from build123d import *

# Parameters (mm, degrees)
SKETCH1_R              = 2.925
SKETCH1_R_2            = 1.75
MIDDLE_RING_DEPTH      = 0.8
SKETCH2_R              = 2.35
SKETCH2_R_2            = 1.75
OUTER_BODY_DEPTH       = 7.35
SKETCH3_R              = 2.625
SKETCH3_R_2            = 1.75
OUTER_RIM_DEPTH        = 0.5
MIDDLE_SLOT_DEPTH      = 9.873204044
MIDDLE_SLOT_DEPTH_BACK = 9.873204044
SIDE_SLOTS_DEPTH       = 9.859105574
SIDE_SLOTS_DEPTH_BACK  = 9.859105574


with BuildPart() as part:
    # Sketch1 → Middle Ring (new, symmetric)
    with BuildSketch(Plane(origin=(0, 0, 0), x_dir=(0, 0, -1), z_dir=(1, 0, 0))):
        Circle(SKETCH1_R)
        Circle(SKETCH1_R_2, mode=Mode.SUBTRACT)
    extrude(amount=MIDDLE_RING_DEPTH, both=True)

    # Sketch2 → Outer Body (add, symmetric)
    with BuildSketch(Plane(origin=(0, 0, 0), x_dir=(0, 0, -1), z_dir=(1, 0, 0))):
        Circle(SKETCH2_R)
        Circle(SKETCH2_R_2, mode=Mode.SUBTRACT)
    extrude(amount=OUTER_BODY_DEPTH, both=True)

    # Sketch3 → Outer Rim (add)
    with BuildSketch(Plane(origin=(7.35, 0, 0), x_dir=(0, 0, -1), z_dir=(1, 0, 0))):
        Circle(SKETCH3_R)
        Circle(SKETCH3_R_2, mode=Mode.SUBTRACT)
    outer_rim = extrude(amount=OUTER_RIM_DEPTH)

    # Mirror1: Outer Rim across plane
    add(outer_rim.mirror(Plane(origin=(0, 0, 0), x_dir=(0, 0, 1), z_dir=(1, 0, 0))))

    # Sketch4 → Middle Slot (cut, two sides: drawn at the far end of the back side and taken through both)
    with BuildSketch(Plane.XY.offset(-MIDDLE_SLOT_DEPTH_BACK)):
        with BuildLine():
            Line((2.95, -0.5), (-2.95, -0.5))
            ThreePointArc((-2.95, -0.5), (-3.45, 0), (-2.95, 0.5))
            Line((-2.95, 0.5), (2.95, 0.5))
            ThreePointArc((2.95, 0.5), (3.45, 0), (2.95, -0.5))
        make_face()
    extrude(amount=MIDDLE_SLOT_DEPTH + MIDDLE_SLOT_DEPTH_BACK, mode=Mode.SUBTRACT)

    # Sketch5 → Side Slots (cut, two sides: drawn at the far end of the back side and taken through both)
    with BuildSketch(Plane(origin=(0, 0, 0), x_dir=(1, 0, 0), z_dir=(0, 1, 0)).offset(-SIDE_SLOTS_DEPTH_BACK)):
        with BuildLine():
            Line((10.95, -0.5), (4.75, -0.5))
            ThreePointArc((4.75, -0.5), (4.25, 0), (4.75, 0.5))
            Line((4.75, 0.5), (10.95, 0.5))
            ThreePointArc((10.95, 0.5), (11.45, 0), (10.95, -0.5))
        make_face()
        with BuildLine():
            Line((-10.95, -0.5), (-4.75, -0.5))
            ThreePointArc((-4.75, -0.5), (-4.25, 0), (-4.75, 0.5))
            Line((-4.75, 0.5), (-10.95, 0.5))
            ThreePointArc((-10.95, 0.5), (-11.45, 0), (-10.95, -0.5))
        make_face()
    extrude(amount=SIDE_SLOTS_DEPTH + SIDE_SLOTS_DEPTH_BACK, mode=Mode.SUBTRACT)


solid = part.part
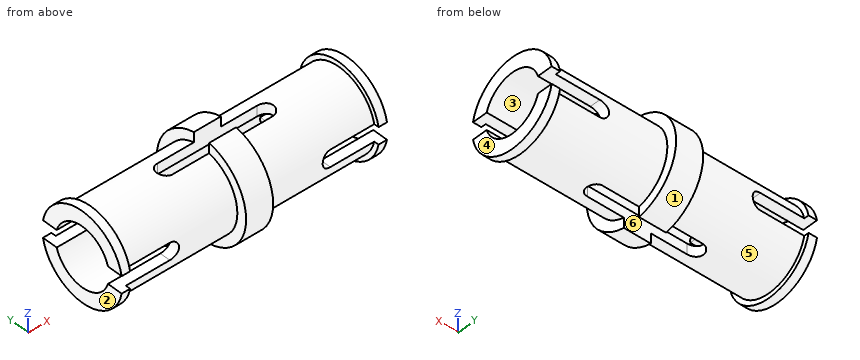
The model under review builds one solid part; all positions refer to its coordinate system, in mm. Face numbers are marked on the shaded views. A direction names the side the tool comes from. Give positions to 0.01 mm unless a question says otherwise; leave off trailing zeros. Loops run counter-clockwise (first coordinate to the right, second up) from the corner with the lowest first, then second, coordinate; pieces in that order, holes last. Notation, with made-up numbers: (49, -25) -> (76, -25) arc R23 cw to (76, 0) -> close; hole circle Ø5 at (71, -26). An arc over 180 degrees is marked (long way). Answer as a JSON object with one key per item and string values. Group by question number.
Q1. Tool access review of the marked faces 4, 5 and 6: name each direction out of +Z, -Z, +X, -X, +Y, -Y from which nothing blocks a thin tool from reaching the whole face with its end or side.
Q2. Draft analysis for pull direction Y (two halves, no side actions). For the marked faces 1, 2 and 3, state which applies: pulls with the +Y half, pulls with the -Y half, needs draft (parallel to the pull), parting line crosses it, or undercut.
Q3. Take a section at C-C (y = 0.2). Write out the cut boundary in (x, z), plus the area to 3 significant figures.
Q4. Take a section at A-A (z = -1.15). Write out the cut boundary in (x, y).
Q5. Take a section at B-B (x = -1.75). Write out the cut boundary in (y, z).
Q6. Insertion check: pin 1 (1.3 mm diameter, centred on x = 1, z = -2, fed in from +Y); pin 2 (0.7 mm diameter, centred on x = 6, y = -2.5, fed in from -Z); pin 3 (1 mm diameter, centred on x = -5.5, y = 2, fed in from +Z); pin 4 (0.6 mm diameter, centred on y = 1, z = 1, fed in from -X). Each pin has a flat end and moves straight along its axis. Give the tip position at first contact, or say it passes through.
Q7. Wall thickness on line 1 along Y through (x, z) = (4, 0); line 2 along X through (y, z) = (-0.3, 2.1): over which ranges is each line inside the solid? List them lowest first.
Q8. Take a section at D-D (y = 1.5). Write out the cut boundary in (x, z).
Answer below:
{
 "1": {"face 4": "+Z, -Z, +X, +Y, -Y", "face 5": "none", "face 6": "+Z, -Z"},
 "2": {"face 1": "pulls with the +Y half", "face 2": "needs draft", "face 3": "undercut"},
 "3": {"outline": "(-7.85, -2.62) -> (-7.35, -2.62) -> (-7.35, -2.34) -> (-3.41, -2.34) -> (-3.41, -1.74) -> (-7.85, -1.74) -> close; (-7.85, 1.74) -> (-3.41, 1.74) -> (-3.41, 2.34) -> (-7.35, 2.34) -> (-7.35, 2.62) -> (-7.85, 2.62) -> close; (3.41, -2.34) -> (7.35, -2.34) -> (7.35, -2.62) -> (7.85, -2.62) -> (7.85, -1.74) -> (3.41, -1.74) -> close; (3.41, 1.74) -> (7.85, 1.74) -> (7.85, 2.62) -> (7.35, 2.62) -> (7.35, 2.34) -> (3.41, 2.34) -> close", "area": "11.3 mm2"},
 "4": {"outline": "(-7.85, -2.36) -> (-7.35, -2.36) -> (-7.35, -2.05) -> (-0.8, -2.05) -> (-0.8, -2.69) -> (0.8, -2.69) -> (0.8, -2.05) -> (7.35, -2.05) -> (7.35, -2.36) -> (7.85, -2.36) -> (7.85, -1.32) -> (-7.85, -1.32) -> close; (-7.85, 1.32) -> (7.85, 1.32) -> (7.85, 2.36) -> (7.35, 2.36) -> (7.35, 2.05) -> (0.8, 2.05) -> (0.8, 2.69) -> (-0.8, 2.69) -> (-0.8, 2.05) -> (-7.35, 2.05) -> (-7.35, 2.36) -> (-7.85, 2.36) -> close"},
 "5": {"outline": "(-0.5, -2.3) -> (-0.5, -1.68) arc R1.75 cw to (-0.5, 1.68) -> (-0.5, 2.3) arc R2.35 ccw to start; (0.5, -2.3) arc R2.35 ccw to (0.5, 2.3) -> (0.5, 1.68) arc R1.75 cw to (0.5, -1.68) -> close"},
 "6": {"pin 1": "stops at y = 2.58", "pin 2": "stops at z = -0.95", "pin 3": "stops at z = 1.81", "pin 4": "passes through"},
 "7": {"line 1": "y = -2.35 to -1.75, 1.75 to 2.35", "line 2": "x = -7.85 to -3.35, 3.35 to 7.85"},
 "8": {"outline": "(-7.85, -2.15) -> (-7.35, -2.15) -> (-7.35, -1.81) -> (-0.8, -1.81) -> (-0.8, -2.51) -> (0.8, -2.51) -> (0.8, -1.81) -> (7.35, -1.81) -> (7.35, -2.15) -> (7.85, -2.15) -> (7.85, -0.9) -> (-7.85, -0.9) -> close; (-7.85, 0.9) -> (7.85, 0.9) -> (7.85, 2.15) -> (7.35, 2.15) -> (7.35, 1.81) -> (0.8, 1.81) -> (0.8, 2.51) -> (-0.8, 2.51) -> (-0.8, 1.81) -> (-7.35, 1.81) -> (-7.35, 2.15) -> (-7.85, 2.15) -> close"}
}
